Model file for the job. Use its own axes, mm. Coordinates: 2 decimals unless noted, no trailing zeros. Write each loop counter-clockwise with the first axis right and the second up, starting at its lowest first coordinate (ties: lowest second). Pieces come first, ordered by that corner, then holes. Notation, with made-up numbers: (-7.5, 51.5) -> (50.5, 51.5) arc R21 cw to (50.5, 74.5) -> close; hole circle Ø9 at (-37.75, 87.5). An arc over 180 degrees is marked (long way). Write item = value, one per line. Start each with the question number.
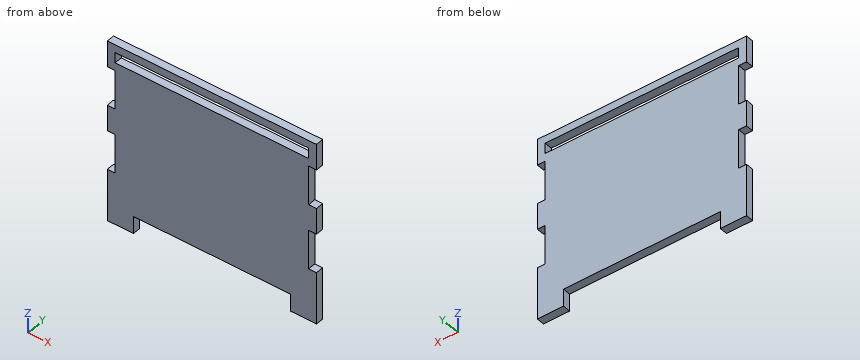
Autodesk Fusion 360 part; units mm, degrees
sketch "Sketch1" plane through (0, 0, 0) normal (0, 0, 1) x (1, 0, 0)
  line L0 (-28.6561, 0.7869) -> (51.3439, 0.7869)
  line L1 (51.3439, 0.7869) -> (51.3439, -2.2131)
  line L2 (51.3439, -2.2131) -> (-28.6561, -2.2131)
  line L3 (-28.6561, -2.2131) -> (-28.6561, 0.7869)
  dimension "d1" = 3
  dimension "d2" = 80
extrude "Extrude1" add sketch "Sketch1" along normal blind 70
sketch "Sketch2" plane through (0, -2.2131, 0) normal (0, -1, 0) x (1, 0, 0)
  line L0 (-28.6561, 0) -> (51.3439, 0)
  line L1 (51.3439, 0) -> (51.3439, 70)
  line L2 (51.3439, 70) -> (-28.6561, 70)
  line L3 (-28.6561, 70) -> (-28.6561, 0)
  line L4 (-18.6561, 0) -> (41.3439, 0)
  line L5 (41.3439, 0) -> (41.3439, 6.61)
  line L6 (41.3439, 6.61) -> (-18.6561, 6.61)
  line L7 (-18.6561, 6.61) -> (-18.6561, 0)
  dimension "d5" = 10
  dimension "d6" = 60
extrude "Extrude2" cut sketch "Sketch2" against normal blind 15 contours L0 L4 L5 L6 L7
sketch "Sketch3" plane through (0, -2.2131, 0) normal (0, -1, 0) x (1, 0, 0)
  line L0 (-18.6561, 0) -> (-18.6561, 6.61)
  line L1 (-18.6561, 6.61) -> (41.3439, 6.61)
  line L2 (41.3439, 6.61) -> (41.3439, 0)
  line L3 (41.3439, 0) -> (51.3439, 0)
  line L4 (51.3439, 0) -> (51.3439, 70)
  line L5 (51.3439, 70) -> (-28.6561, 70)
  line L6 (-28.6561, 70) -> (-28.6561, 0)
  line L7 (-28.6561, 0) -> (-18.6561, 0)
  line L8 (59.8727, 60) -> (-42.4062, 60) construction
  line L9 (-42.8479, 45) -> (61.1574, 45) construction
  line L10 (63.7389, 35) -> (-40.2664, 35) construction
  line L11 (-40.2664, 20) -> (63.7389, 20) construction
  line L12 (48.3439, -12.0113) -> (48.3439, -4.8877)
  line L13 (48.3439, -4.8877) -> (48.3439, 80.5961) construction
  line L14 (-25.6561, 80.5961) -> (-25.6561, -19.135) construction
  line L15 (-25.6561, 60) -> (-28.6561, 60)
  line L16 (-28.6561, 60) -> (-28.6561, 45)
  line L17 (-28.6561, 45) -> (-25.6561, 45)
  line L18 (-25.6561, 45) -> (-25.6561, 60)
  line L19 (-25.6561, 35) -> (-28.6561, 35)
  line L20 (-28.6561, 35) -> (-28.6561, 20)
  line L21 (-28.6561, 20) -> (-25.6561, 20)
  line L22 (-25.6561, 20) -> (-25.6561, 35)
  line L23 (48.3439, 20) -> (51.3439, 20)
  line L24 (51.3439, 20) -> (51.3439, 35)
  line L25 (51.3439, 35) -> (48.3439, 35)
  line L26 (48.3439, 35) -> (48.3439, 20)
  line L27 (48.3439, 45) -> (51.3439, 45)
  line L28 (51.3439, 45) -> (51.3439, 60)
  line L29 (51.3439, 60) -> (48.3439, 60)
  line L30 (48.3439, 60) -> (48.3439, 45)
  line L31 (-25.6561, 67) -> (48.3439, 67)
  line L32 (48.3439, 67) -> (48.3439, 63)
  line L33 (48.3439, 63) -> (-25.6561, 63)
  line L34 (-25.6561, 63) -> (-25.6561, 67)
  dimension "d9" = 3
  dimension "d10" = 3
  dimension "d11" = 10
  dimension "d12" = 15
  dimension "d13" = 10
  dimension "d14" = 15
  dimension "d17" = 4
  dimension "d18" = 3
extrude "Extrude3" cut sketch "Sketch3" against normal blind 10 contours L6 L19 L20 L21 L22 | L6 L15 L16 L17 L18 | L4 L23 L24 L25 L26 | L4 L27 L28 L29 L30 | L31 L32 L33 L34
(1) Saw through at A-A (x = 28.5). Give the cut face in (y, z).
(2) Saw through at C-C (z = 33). Give the cut face in (x, y).
(3) Saw through at B-B (y = -1.4). Give the cut face in (x, z).
(4) Drill centre lines: line 1 along Z through (x, y) = (1.5, -0.65); line 2 along Z through (x, y) = (44, -1.15); line 3 along X through (y, z) = (-0.45, 46). Where is each one in solid material? Low to high.
(5) Drop flat-ended pins along their axis: pin 1 Ø0.9 at (x, y) = (28, -1.5) entering from -Z; pin 2 Ø1.5 at (x, y) = (49.5, -1) entering from -Z. Give the stop position or say it passes through.
Returned:
q1.outline = (-2.21, 6.61) -> (0.79, 6.61) -> (0.79, 63) -> (-2.21, 63) -> close; (-2.21, 67) -> (0.79, 67) -> (0.79, 70) -> (-2.21, 70) -> close
q2.outline = (-25.66, -2.21) -> (48.34, -2.21) -> (48.34, 0.79) -> (-25.66, 0.79) -> close
q3.outline = (-28.66, 0) -> (-18.66, 0) -> (-18.66, 6.61) -> (41.34, 6.61) -> (41.34, 0) -> (51.34, 0) -> (51.34, 20) -> (48.34, 20) -> (48.34, 35) -> (51.34, 35) -> (51.34, 45) -> (48.34, 45) -> (48.34, 60) -> (51.34, 60) -> (51.34, 70) -> (-28.66, 70) -> (-28.66, 60) -> (-25.66, 60) -> (-25.66, 45) -> (-28.66, 45) -> (-28.66, 35) -> (-25.66, 35) -> (-25.66, 20) -> (-28.66, 20) -> close; hole (-25.66, 63) -> (48.34, 63) -> (48.34, 67) -> (-25.66, 67) -> close
q4.line_1 = 6.61 to 63, 67 to 70
q4.line_2 = 0 to 63, 67 to 70
q4.line_3 = -25.66 to 48.34
q5.pin_1 = 6.61
q5.pin_2 = 0
